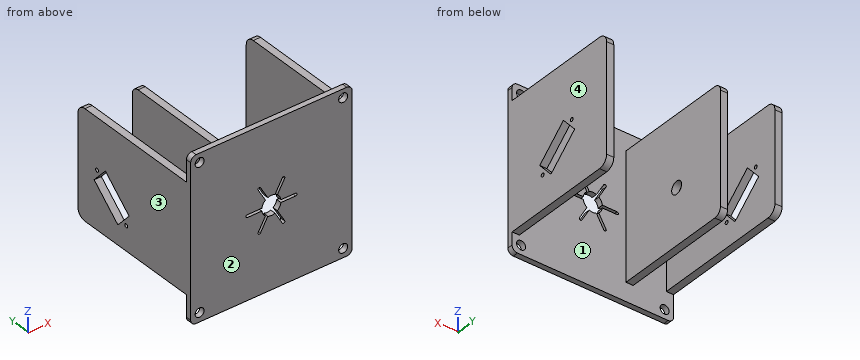
from build123d import *

# Parameters (mm, degrees)
SKETCH1_W           = 4
SKETCH1_H           = 70
SKETCH1_H_2         = 60
BOSS_EXTRUDE1_DEPTH = 3
SKETCH1_3_W         = 4
SKETCH1_3_H         = 60
SKETCH1_3_H_2       = 70
BOSS_EXTRUDE2_DEPTH = 70
SKETCH1_4_W         = 4
SKETCH1_4_H         = 70
BOSS_EXTRUDE3_DEPTH = 70
SKETCH5_R           = 4
CUT_EXTRUDE4_DEPTH  = 10
SKETCH6_R           = 2.5
CUT_EXTRUDE5_DEPTH  = 10
SKETCH1_5_W         = 4
SKETCH1_5_H         = 60
BOSS_EXTRUDE4_DEPTH = 80
SKETCH5_2_R         = 4
CUT_EXTRUDE6_DEPTH  = 10
FILLET1_R           = 3
FILLET2_R           = 5
FILLET3_R           = 4
SKETCH7_R           = 2.5
CUT_EXTRUDE7_DEPTH  = 10
SKETCH8_R           = 2.5
CUT_EXTRUDE8_DEPTH  = 10
CUT_EXTRUDE9_REACH  = 132.084
SKETCH9_R           = 3.5
SKETCH26_R          = 2.5
CUT_EXTRUDE11_DEPTH = 10
CUT_EXTRUDE14_DEPTH = 10
CUT_EXTRUDE15_DEPTH = 10
SKETCH28_R          = 1
SKETCH28_R_2        = 4
CUT_EXTRUDE16_DEPTH = 4
SKETCH29_R          = 1
SKETCH29_R_2        = 3.5
CUT_EXTRUDE18_DEPTH = 4
SKETCH31_R          = 5.375
CUT_EXTRUDE19_DEPTH = 10


with BuildPart() as part:
    # Sketch1 → Boss-Extrude1 (new body)
    # profile 1 of 4: a face of its own
    with BuildSketch(Plane(origin=(0, 0, 0), x_dir=(1, 0, 0), z_dir=(0, 1, 0))):
        Polygon((-50.771305032, 49.212548619), (-50.771305032, 34.212548619), (-46.771305032, 34.212548619), (-46.771305032, -25.787451381), (-50.771305032, -25.787451381), (-50.771305032, -40.787451381), (39.228694968, -40.787451381), (39.228694968, -30.787451381), (35.228694968, -30.787451381), (35.228694968, 39.212548619), (39.228694968, 39.212548619), (39.228694968, 49.212548619), align=None)
        with Locations((-26.271305032, 3.893815937)):
            Rectangle(SKETCH1_W, SKETCH1_H, mode=Mode.SUBTRACT)
    # profile 2 of 4: a face of its own
    with BuildSketch(Plane(origin=(0, 0, 0), x_dir=(1, 0, 0), z_dir=(0, 1, 0))):
        with Locations((37.228694968, 4.212548619)):
            Rectangle(SKETCH1_W, SKETCH1_H)
    # profile 3 of 4: a face of its own
    with BuildSketch(Plane(origin=(0, 0, 0), x_dir=(1, 0, 0), z_dir=(0, 1, 0))):
        with Locations((-48.771305032, 4.212548619)):
            Rectangle(SKETCH1_W, SKETCH1_H_2)
    # profile 4 of 4: a face of its own
    with BuildSketch(Plane(origin=(0, 0, 0), x_dir=(1, 0, 0), z_dir=(0, 1, 0))):
        with Locations((-26.271305032, 3.893815937)):
            Rectangle(SKETCH1_W, SKETCH1_H)
    extrude(amount=BOSS_EXTRUDE1_DEPTH)

    # Sketch1<3> → Boss-Extrude2 (add)
    with BuildSketch(Plane(origin=(0, 0, 0), x_dir=(1, 0, 0), z_dir=(0, 1, 0))):
        with Locations((-48.771305032, 4.212548619)):
            Rectangle(SKETCH1_3_W, SKETCH1_3_H)
        with Locations((37.228694968, 4.212548619)):
            Rectangle(SKETCH1_3_W, SKETCH1_3_H_2)
    extrude(amount=BOSS_EXTRUDE2_DEPTH)

    # Sketch1<4> → Boss-Extrude3 (add)
    with BuildSketch(Plane(origin=(0, 0, 0), x_dir=(1, 0, 0), z_dir=(0, 1, 0))):
        with Locations((-26.271305032, 3.893815937)):
            Rectangle(SKETCH1_4_W, SKETCH1_4_H)
    extrude(amount=BOSS_EXTRUDE3_DEPTH)

    # Sketch5 → Cut-Extrude4 (cut)
    with BuildSketch(Plane.ZY.offset(50.771305032)):
        with Locations((-8.022548619, 60)):
            Circle(SKETCH5_R)
    extrude(amount=-CUT_EXTRUDE4_DEPTH, mode=Mode.SUBTRACT)

    # Sketch6 → Cut-Extrude5 (cut)
    with BuildSketch(Plane(origin=(0, 3, 0), x_dir=(1, 0, 0), z_dir=(0, 1, 0))):
        with Locations(Location((-45.787574368, -35.787451381, 0), (0, 0, 270))):
            Circle(SKETCH6_R)
        with Locations(Location((-45.787574368, 44.212548619, 0), (0, 0, 270))):
            Circle(SKETCH6_R)
        with Locations((43.718511914, 44.212548619)):
            Circle(SKETCH6_R)
        with Locations((43.718511914, -35.787451381)):
            Circle(SKETCH6_R)
    extrude(amount=-CUT_EXTRUDE5_DEPTH, mode=Mode.SUBTRACT)

    # Sketch1<5> → Boss-Extrude4 (add)
    with BuildSketch(Plane(origin=(0, 0, 0), x_dir=(1, 0, 0), z_dir=(0, 1, 0))):
        with Locations((-48.771305032, 4.212548619)):
            Rectangle(SKETCH1_5_W, SKETCH1_5_H)
    extrude(amount=BOSS_EXTRUDE4_DEPTH)

    # Sketch5<2> → Cut-Extrude6 (cut)
    with BuildSketch(Plane.ZY.offset(50.771305032)):
        with Locations((-8.022548619, 60)):
            Circle(SKETCH5_2_R)
    extrude(amount=-CUT_EXTRUDE6_DEPTH, mode=Mode.SUBTRACT)

    # Fillet1
    fillet1_edges = [part.edges().sort_by_distance(p)[0] for p in [
        (-50.771305032, 1.5, 40.787451381),
        (-50.771305032, 1.5, -49.212548619),
        (39.228694968, 1.5, -49.212548619),
        (39.228694968, 1.5, 40.787451381),
    ]]
    fillet(fillet1_edges, radius=FILLET1_R)

    # Fillet2
    fillet2_edges = [part.edges().sort_by_distance(p)[0] for p in [
        (-48.771305032, 80, -34.212548619),
        (-48.771305032, 80, 25.787451381),
        (37.228694968, 70, -39.212548619),
        (37.228694968, 70, 30.787451381),
    ]]
    fillet(fillet2_edges, radius=FILLET2_R)

    # Fillet3
    fillet3_edges = [part.edges().sort_by_distance(p)[0] for p in [
        (-26.271305032, 70, 31.106184063),
        (-26.271305032, 70, -38.893815937),
    ]]
    fillet(fillet3_edges, radius=FILLET3_R)

    # Sketch7 → Cut-Extrude7 (cut)
    with BuildSketch(Plane(origin=(39.228694968, 0, 0), x_dir=(0, 0, -1), z_dir=(1, 0, 0))):
        with Locations((27.482306935, -10)):
            Circle(SKETCH7_R)
    extrude(amount=-CUT_EXTRUDE7_DEPTH, mode=Mode.SUBTRACT)

    # Sketch8 → Cut-Extrude8 (cut)
    with BuildSketch(Plane(origin=(39.228694968, 0, 0), x_dir=(0, 0, -1), z_dir=(1, 0, 0))):
        with Locations((8.02072759, 38.893893193)):
            Circle(SKETCH8_R)
    extrude(amount=-CUT_EXTRUDE8_DEPTH, mode=Mode.SUBTRACT)

    # Cut-Extrude9: up to this face of the body (flat: up to its plane)
    cut_extrude9_end = Plane(part.part.faces().sort_by_distance((-28.271305032, 36.452186393, -3.893815937))[0])
    # Sketch9 → Cut-Extrude9 (cut, up to the picked face)
    with BuildSketch(Plane(origin=(39.228694968, 0, 0), x_dir=(0, 0, -1), z_dir=(1, 0, 0)), mode=Mode.PRIVATE) as cut_extrude9_sk1:
        with Locations((8.02072759, 38.893893193)):
            Circle(SKETCH9_R)
    cut_extrude9_tool1 = split(extrude(cut_extrude9_sk1.sketch, amount=-CUT_EXTRUDE9_REACH, mode=Mode.PRIVATE), bisect_by=cut_extrude9_end, keep=Keep.BOTH, mode=Mode.PRIVATE)
    add(cut_extrude9_tool1.solids().sort_by(Axis((39.228695, 38.893893, -8.020728), (-1, 0, 0)))[0], mode=Mode.SUBTRACT)

    # Sketch26 → Cut-Extrude11 (cut)
    with BuildSketch(Plane(origin=(0, 3, 0), x_dir=(1, 0, 0), z_dir=(0, 1, 0))):
        with Locations(Location((34.228694968, -36.063353705, 0), (0, 0, 270))):
            Circle(SKETCH26_R)
        with Locations(Location((34.228694968, 44.212548619, 0), (0, 0, 270))):
            Circle(SKETCH26_R)
    extrude(amount=-CUT_EXTRUDE11_DEPTH, mode=Mode.SUBTRACT)

    # Sketch27 → Cut-Extrude14 (cut)
    with BuildSketch(Plane(origin=(0, 3, 0), x_dir=(1, 0, 0), z_dir=(0, 1, 0))):
        with BuildLine():
            Line((7.728694968, 3.462548619), (-19.271305032, 3.462548619))
            ThreePointArc((-19.271305032, 3.462548619), (-20.021305032, 4.212548619), (-19.271305032, 4.962548619))
            Line((-19.271305032, 4.962548619), (7.728694968, 4.962548619))
            ThreePointArc((7.728694968, 4.962548619), (8.478694968, 4.212548619), (7.728694968, 3.462548619))
        make_face()
        with BuildLine():
            Line((0.329175915, -7.853794332), (-13.170824085, 15.52889157))
            ThreePointArc((-13.170824085, 15.52889157), (-12.896305032, 16.553410623), (-11.871785979, 16.27889157))
            Line((-11.871785979, 16.27889157), (1.628214021, -7.103794332))
            ThreePointArc((1.628214021, -7.103794332), (1.353694968, -8.128313385), (0.329175915, -7.853794332))
        make_face()
        with BuildLine():
            Line((-13.170824085, -7.103794332), (0.329175915, 16.27889157))
            ThreePointArc((0.329175915, 16.27889157), (1.353694968, 16.553410623), (1.628214021, 15.52889157))
            Line((1.628214021, 15.52889157), (-11.871785979, -7.853794332))
            ThreePointArc((-11.871785979, -7.853794332), (-12.896305032, -8.128313385), (-13.170824085, -7.103794332))
        make_face()
    extrude(amount=-CUT_EXTRUDE14_DEPTH, mode=Mode.SUBTRACT)

    # Sketch27<7> → Cut-Extrude15 (cut)
    with BuildSketch(Plane(origin=(0, 3, 0), x_dir=(1, 0, 0), z_dir=(0, 1, 0))):
        with BuildLine():
            Line((-7.743699741, 2.296260771), (-7.070343138, 3.462548619))
            Line((-7.070343138, 3.462548619), (-8.417056343, 3.462548619))
            ThreePointArc((-8.417056343, 3.462548619), (-8.152874893, 2.837548619), (-7.743699741, 2.296260771))
        make_face()
        with BuildLine():
            Line((-8.417056343, 4.962548619), (-7.070343138, 4.962548619))
            Line((-7.070343138, 4.962548619), (-7.743699741, 6.128836466))
            ThreePointArc((-7.743699741, 6.128836466), (-8.152874893, 5.587548619), (-8.417056343, 4.962548619))
        make_face()
        with BuildLine():
            Line((-5.771305032, 5.712548619), (-5.09794843, 6.878836466))
            ThreePointArc((-5.09794843, 6.878836466), (-5.771305032, 6.962548619), (-6.444661635, 6.878836466))
            Line((-6.444661635, 6.878836466), (-5.771305032, 5.712548619))
        make_face()
        with BuildLine():
            Line((-4.472266927, 4.962548619), (-3.125553721, 4.962548619))
            ThreePointArc((-3.125553721, 4.962548619), (-3.389735172, 5.587548619), (-3.798910324, 6.128836466))
            Line((-3.798910324, 6.128836466), (-4.472266927, 4.962548619))
        make_face()
        with BuildLine():
            ThreePointArc((-3.798910324, 2.296260771), (-3.389735172, 2.837548619), (-3.125553721, 3.462548619))
            Line((-3.125553721, 3.462548619), (-4.472266927, 3.462548619))
            Line((-4.472266927, 3.462548619), (-3.798910324, 2.296260771))
        make_face()
        with BuildLine():
            ThreePointArc((-6.444661635, 1.546260771), (-5.771305032, 1.462548619), (-5.09794843, 1.546260771))
            Line((-5.09794843, 1.546260771), (-5.771305032, 2.712548619))
            Line((-5.771305032, 2.712548619), (-6.444661635, 1.546260771))
        make_face()
    extrude(amount=-CUT_EXTRUDE15_DEPTH, mode=Mode.SUBTRACT)

    # Sketch28 → Cut-Extrude16 (cut)
    # profile 1 of 3: a face of its own
    with BuildSketch(Plane.ZY.offset(50.771305032)):
        with Locations((-2.316893756, 66.434710762)):
            Circle(SKETCH28_R)
    # profile 2 of 3: a face of its own
    with BuildSketch(Plane.ZY.offset(50.771305032)):
        with Locations((-20.69441, 45.708956331)):
            Circle(SKETCH28_R)
    # profile 3 of 3: a face of its own
    with BuildSketch(Plane.ZY.offset(50.771305032)):
        Polygon((-23.458777666, 51.635023443), (-8.531192269, 68.470022529), (0.44747391, 60.508643651), (-14.480111487, 43.673644564), align=None)
        with Locations((-8.022548619, 60)):
            Circle(SKETCH28_R_2, mode=Mode.SUBTRACT)
    extrude(amount=-CUT_EXTRUDE16_DEPTH, mode=Mode.SUBTRACT)

    # Sketch29 → Cut-Extrude18 (cut)
    # profile 1 of 3: a face of its own
    with BuildSketch(Plane(origin=(39.228694968, 0, 0), x_dir=(0, 0, -1), z_dir=(1, 0, 0))):
        with Locations((2.315072727, 45.328603955)):
            Circle(SKETCH29_R)
    # profile 2 of 3: a face of its own
    with BuildSketch(Plane(origin=(39.228694968, 0, 0), x_dir=(0, 0, -1), z_dir=(1, 0, 0))):
        with Locations((20.692588971, 24.602849525)):
            Circle(SKETCH29_R)
    # profile 3 of 3: a face of its own
    with BuildSketch(Plane(origin=(39.228694968, 0, 0), x_dir=(0, 0, -1), z_dir=(1, 0, 0))):
        Polygon((8.529371241, 47.363915722), (23.456956637, 30.528916636), (14.478290458, 22.567537758), (-0.449294939, 39.402536844), align=None)
        with Locations((8.02072759, 38.893893193)):
            Circle(SKETCH29_R_2, mode=Mode.SUBTRACT)
    extrude(amount=-CUT_EXTRUDE18_DEPTH, mode=Mode.SUBTRACT)

    # Sketch31 → Cut-Extrude19 (cut)
    with BuildSketch(Plane(origin=(0, 3, 0), x_dir=(1, 0, 0), z_dir=(0, 1, 0))):
        with Locations((-5.771305032, 4.212548619)):
            Circle(SKETCH31_R)
    extrude(amount=-CUT_EXTRUDE19_DEPTH, mode=Mode.SUBTRACT)


solid = part.part
The listing builds one solid part. Answer for the finished solid, in the listing's coordinates (mm). Face numbers are marked on the shaded views. Coordinates: 2 decimals unless noted, no trailing zeros. Order: outer loops, then holes, each group sorted by start corner. A loop starts at its lowest first (then second) coordinate and runs counter-clockwise, first axis right, second up. Notation, with made-up numbers: M -14.75,66.5 L 5.25,66.5 A23 cw 5.25,89.5 Z; hole C -28.5,-14.5 d5. An arc over 180 degrees is marked long. Use CSV: the item, a comma, the result in double quotes.
Q1. Section C-C (z = 14) is taken. Determine the outline of the cut face in (x, y).
Here are the results:
outline,"M -50.77,0 L 39.23,0 L 39.23,70 L 35.23,70 L 35.23,3 L -24.27,3 L -24.27,70 L -28.27,70 L -28.27,3 L -46.77,3 L -46.77,80 L -50.77,80 Z"
Q2. Given pin 1 Ø2.5 at (y, z) = (45.33, -2.32) entering from +X; pin 2 Ø1.2 at (x, y) = (36.5, 29) entering from -Z; pin 3 Ø4.5 at (x, y) = (-25.5, 27) entering from -Z; pin 4 Ø4.5 at (x, y) = (-26.5, 20) entering from +Z, each flat-ended and moving along its own axis, determine where each tip first touches the part or whether it passes through.
Here are the results:
pin 1,"x = 39.23"
pin 2,"z = -39.21"
pin 3,"z = -38.89"
pin 4,"z = 31.11"
Q3. Section D-D (x = -39.5) is taken. Determine the outline of the cut face in (y, z).
Here are the results:
outline,"M 0,-49.21 L 3,-49.21 L 3,40.79 L 0,40.79 Z"
Q4. Straight lines are drawn through the part: L1, parallel to X at y = 43, z = 7; L2, parallel to X at y = 62, z = -8.5; L3, parallel to Y at x = -43.5, z = -24.5. For each, find the intervals that lie inside material, in ascending order.
Here are the results:
L1,"-50.77 to -46.77, -28.27 to -24.27, 35.23 to 39.23"
L2,"-28.27 to -24.27, 35.23 to 39.23"
L3,"0 to 3"
Q5. Determine the mould class of the marked faces 1, 2, 3 and 4 for opening direction X: pulls with the +X half, pulls with the -X half, needs draft (parallel to the pull), parting line crosses it, or undercut.
Here are the results:
face 1,"undercut"
face 2,"needs draft"
face 3,"pulls with the -X half"
face 4,"pulls with the +X half"
Q6. Section A-A (y = 18) is taken. Determine the outline of the cut face in (x, z), then the cut area to 3 significant figures.
Here are the results:
outline,"M -50.77,-34.21 L -46.77,-34.21 L -46.77,25.79 L -50.77,25.79 Z; M -28.27,-38.89 L -24.27,-38.89 L -24.27,31.11 L -28.27,31.11 Z; M 35.23,-39.21 L 39.23,-39.21 L 39.23,30.79 L 35.23,30.79 Z"
area,"800 mm2"
Q7. Section B-B (y = 62.5) is taken. Determine the outline of the cut face in (x, z), then the cut area to 3 significant figures.
Here are the results:
outline,"M -50.77,-34.21 L -46.77,-34.21 L -46.77,-13.82 L -50.77,-13.82 Z; M -50.77,-1.8 L -46.77,-1.8 L -46.77,25.79 L -50.77,25.79 Z; M -28.27,-38.89 L -24.27,-38.89 L -24.27,31.11 L -28.27,31.11 Z; M 35.23,-39.21 L 39.23,-39.21 L 39.23,30.79 L 35.23,30.79 Z"
area,"752 mm2"
